For this review, take the finished solid that the model builds, in its own axes (mm). A direction names the side the tool comes from. Coordinates: 2 decimals unless noted, no trailing zeros. Order: outer loops, then holes, each group sorted by start corner. A loop starts at its lowest first (then second) coordinate and runs counter-clockwise, first axis right, second up.
from build123d import *

# Parameters (mm, degrees)
BOSS_EXTRU_1_DEPTH      = 6
ESQUISSE2_R             = 1.5
ENL_V_MAT_EXTRU_1_DEPTH = 6
ESQUISSE3_R             = 2.995
ENL_V_MAT_EXTRU_2_DEPTH = 3


with BuildPart() as part:
    # Esquisse1 → Boss.-Extru.1 (new body)
    with BuildSketch(Plane.XY):
        Polygon((-47.5, 78), (-80, 78), (-80, 0), (-47.5, 0), (-47.5, -6), (-32.5, -6), (-32.5, 0), (0, 0), (0, 78), (-32.5, 78), (-32.5, 84), (-47.5, 84), align=None)
    extrude(amount=BOSS_EXTRU_1_DEPTH)

    # Esquisse2 → Enlèv. mat.-Extru.1 (cut)
    with BuildSketch(Plane(origin=(0, 0, 0), x_dir=(-1, 0, 0), z_dir=(0, 0, -1))):
        with Locations((40, 81)):
            Circle(ESQUISSE2_R)
    extrude(amount=-ENL_V_MAT_EXTRU_1_DEPTH, mode=Mode.SUBTRACT)

    # Esquisse3 → Enlèv. mat.-Extru.2 (cut)
    with BuildSketch(Plane(origin=(0, 0, 0), x_dir=(-1, 0, 0), z_dir=(0, 0, -1))):
        with Locations((40, 81)):
            Circle(ESQUISSE3_R)
    extrude(amount=-ENL_V_MAT_EXTRU_2_DEPTH, mode=Mode.SUBTRACT)


solid = part.part
1. Clearance check with flat-ended pins moving along their axes: pin 1 Ø1.8 at (y, z) = (-4.5, 3) entering from -X; pin 2 Ø1.8 at (y, z) = (-2.5, 3) entering from +X; pin 3 Ø1.8 at (x, z) = (-14.5, 4.5) entering from -Y. State where each tip first meets the part, or that it passes through.
Answer below:
pin 1: stops at x = -47.5
pin 2: stops at x = -32.5
pin 3: stops at y = 0
2. Take a section at D-D, the plane x = -63. Give the boundary of the cut face in (y, z).
Answer below:
outline: (0, 0) - (78, 0) - (78, 6) - (0, 6) - close
3. To check wall thickness, follow L1, parallel to Y at x = -40, z = 4.65; L2, parallel to X at y = 81, z = 5.35; L3, parallel to X at y = -1.5, z = 1.2. State the ranges of each line that lie inside material, in increasing order.
Answer below:
L1: y = -6 to 79.5, 82.5 to 84
L2: x = -47.5 to -41.5, -38.5 to -32.5
L3: x = -47.5 to -32.5
4. Take a section at B-B, the plane y = 81. Give the boundary of the cut face in (x, z) (3 decimals).
Answer below:
outline: (-47.5, 0) - (-42.995, 0) - (-42.995, 3) - (-41.5, 3) - (-41.5, 6) - (-47.5, 6) - close; (-38.5, 3) - (-37.005, 3) - (-37.005, 0) - (-32.5, 0) - (-32.5, 6) - (-38.5, 6) - close
5. Take a section at C-C, the plane x = -40. Give the boundary of the cut face in (y, z) (3 decimals), plus the area to 3 significant figures.
Answer below:
outline: (-6, 0) - (78.005, 0) - (78.005, 3) - (79.5, 3) - (79.5, 6) - (-6, 6) - close; (82.5, 3) - (83.995, 3) - (83.995, 0) - (84, 0) - (84, 6) - (82.5, 6) - close
area: 513 mm2
6. Take a section at A-A, the plane z = 2. Give the boundary of the cut face in (x, y) (3 decimals), plus the area to 3 significant figures.
Answer below:
outline: (-80, 0) - (-47.5, 0) - (-47.5, -6) - (-32.5, -6) - (-32.5, 0) - (0, 0) - (0, 78) - (-32.5, 78) - (-32.5, 84) - (-47.5, 84) - (-47.5, 78) - (-80, 78) - close; hole circle Ø5.99 at (-40, 81)
area: 6,390 mm2
7. The part is to be moulded in two halves that separate along Y. For faces 6 (the face through (-64, 78, 3)), 7 (the face through (-39.805, 82.487, 4.479)), 8 (the face through (0, 38, 3)), 9 (the face through (-40, -6, 3)), say which applies: +Y half, -Y half, draft (parallel to the pull), parting line (faces both ways), or undercut.
Answer below:
face 6: +Y half
face 7: undercut
face 8: draft
face 9: -Y half
8. Machinability: for faces 1 (the face through (-47.5, -3, 3)), 2 (the face through (-42.767, 79.853, 1.479)), 3 (the face through (-32.5, 81, 3)), 4 (the face through (-47.5, 81, 3)), 5 (the face through (-16, 0, 3)), which of the approach directions +Z, -Z, +X, -X, +Y, -Y give a long, thin tool a straight path to every point of the face, cutting with its end or side? Answer none if there is none.
Answer below:
face 1: +Z, -Z, -X, -Y
face 2: -Z
face 3: +Z, -Z, +X, +Y
face 4: +Z, -Z, -X, +Y
face 5: +Z, -Z, +X, -Y
